Here's how the part is built. I have some questions about the finished solid (model axes, mm). Round coordinates to 2 decimals unless told otherwise and drop trailing zeros. Order: outer loops, then holes, each group sorted by start corner. A loop starts at its lowest first (then second) coordinate and runs counter-clockwise, first axis right, second up.
```python
from build123d import *

# Parameters (mm, degrees)
F0_W         = 73.972383514
F0_H         = 1.5005278401
F1_DEPTH     = 3.25
F2_R         = 1.375
F3_R         = 1.375
F4_T1_DEPTH  = 42.9737045288
F4_T3_DEPTH  = 0.5
F4_T5_DEPTH  = 97.1535263256
F4_T10_DEPTH = 1.375
F4_T16_DEPTH = 1.375
F4_T20_ANGLE = 62.6710528925
F4_T22_ANGLE = 62.6710528925


# Not quite as in the source:
# - a fillet or chamfer that OpenCascade refuses, or shapes differently, is made with other operations: its cross-section is extruded or revolved along the edge and cut away or added


with BuildPart() as f1:
    # F0 (on Top) → F1 (new body)
    with BuildSketch(Plane.XY):
        with BuildLine():
            Line((62.3850544982, 0), (62.3850544982, 8.25))
            Line((62.3850544982, 8.25), (-31.3309718274, 8.25))
            ThreePointArc((-31.3309718274, 8.25), (-35.6733794922, 7.0320400779), (-38.7489899112, 3.7334720175))
            Line((-38.7489899112, 3.7334720175), (-59.5149430004, -36.45))
            Line((-59.5149430004, -36.45), (-57.0939640871, -36.45))
            ThreePointArc((-57.0939640871, -36.45), (-52.4551081593, -35.0428751739), (-49.3797131513, -31.2957522588))
            Line((-49.3797131513, -31.2957522588), (-38.5501753509, -5.1542477412))
            ThreePointArc((-38.5501753509, -5.1542477412), (-35.474780343, -1.4071248261), (-30.8359244151, 0))
            Line((-30.8359244151, 0), (62.3850544982, 0))
        make_face()
        with Locations((14.1874579713, 4.9997360799)):
            Rectangle(F0_W, F0_H, mode=Mode.SUBTRACT)
    extrude(amount=F1_DEPTH)

    # F2
    f2_edges = [f1.edges().sort_by_distance(p)[0] for p in [
        (15.774565, 0, 3.25),
    ]]
    fillet(f2_edges, radius=F2_R)

    # F3
    f3_edges = [f1.edges().sort_by_distance(p)[0] for p in [
        (15.774565, 0, 0),
    ]]
    fillet(f3_edges, radius=F3_R)

    # F4: fillet of radius 1.375 on 2 edges, made by hand

    # F4_s2 → F4_t1 (cut)
    with BuildSketch(Plane(origin=(-6.6444578792, -12.8574588468, 0), x_dir=(0, 0, 1), z_dir=(-0.4590984452, -0.8883853993, 0))):
        with BuildLine():
            ThreePointArc((1.375, 36.1380680715), (0.4027281759, 35.7353398956), (0, 34.7630680715))
            Line((0, 34.7630680715), (0, 36.1380680715))
            Line((0, 36.1380680715), (1.375, 36.1380680715))
        make_face()
        with BuildLine():
            ThreePointArc((1.875, 36.1380680715), (2.8472718241, 35.7353398956), (3.25, 34.7630680715))
            Line((3.25, 34.7630680715), (3.25, 36.1380680715))
            Line((3.25, 36.1380680715), (1.875, 36.1380680715))
        make_face()
    extrude(amount=F4_T1_DEPTH, mode=Mode.SUBTRACT)

    # F4_s4 → F4_t3 (cut)
    with BuildSketch(Plane.XY.offset(1.375)):
        with BuildLine():
            ThreePointArc((-58.478150845, -34.4437396378), (-58.4310586584, -35.7900671304), (-57.256620921, -36.45))
            Line((-57.256620921, -36.45), (-59.5149430004, -36.45))
            Line((-59.5149430004, -36.45), (-58.478150845, -34.4437396378))
        make_face()
    extrude(amount=F4_T3_DEPTH, mode=Mode.SUBTRACT)

    # F4_s6 → F4_t5 (cut)
    with BuildSketch(Plane.YZ.offset(-31.3309718274)):
        with BuildLine():
            ThreePointArc((6.875, 3.25), (7.8472718241, 2.8472718241), (8.25, 1.875))
            Line((8.25, 1.875), (8.25, 3.25))
            Line((8.25, 3.25), (6.875, 3.25))
        make_face()
        with BuildLine():
            ThreePointArc((6.875, 0), (7.8472718241, 0.4027281759), (8.25, 1.375))
            Line((8.25, 1.375), (8.25, 0))
            Line((8.25, 0), (6.875, 0))
        make_face()
    extrude(amount=F4_T5_DEPTH, mode=Mode.SUBTRACT)


with BuildPart() as f4_tool8:
    # F4_s9 → F4_t10 (new body)
    with BuildSketch(Plane.XY.offset(1.875)):
        Polygon((-57.256620921, -35.075), (-58.478150845, -34.4437396378), (-59.5149430004, -36.45), (-57.256620921, -36.45), align=None)
    extrude(amount=F4_T10_DEPTH)

    # F4_s11 → F4_t12 (revolve, cut)
    with BuildSketch(Plane(origin=(-57.256620921, -35.075, 1.875), x_dir=(0.8541365363, 0.5200488221, 0), z_dir=(0.5200488221, -0.8541365363, 0))):
        with BuildLine():
            ThreePointArc((0, -1.375), (1.375, 0), (0, 1.375))
            Line((0, 1.375), (0, -1.375))
        make_face()
    revolve(axis=Axis((-57.256620921, -35.075, 1.875), (0, 0, 1)), mode=Mode.SUBTRACT)


with BuildPart() as f1_1:
    add(f1.part)

    # F4_t7: cut F4_tool8
    add(f4_tool8.part, mode=Mode.SUBTRACT)


with BuildPart() as f4_tool14:
    # F4_s15 → F4_t16 (new body)
    with BuildSketch(Plane.XY.offset(1.375)):
        Polygon((-57.256620921, -35.075), (-58.478150845, -34.4437396378), (-59.5149430004, -36.45), (-57.256620921, -36.45), align=None)
    extrude(amount=-F4_T16_DEPTH)

    # F4_s17 → F4_t18 (revolve, cut)
    with BuildSketch(Plane(origin=(-57.256620921, -35.075, 1.375), x_dir=(0.8541365363, 0.5200488221, 0), z_dir=(-0.5200488221, 0.8541365363, 0))):
        with BuildLine():
            ThreePointArc((0, -1.375), (1.375, 0), (0, 1.375))
            Line((0, 1.375), (0, -1.375))
        make_face()
    revolve(axis=Axis((-57.256620921, -35.075, 1.375), (0, 0, -1)), mode=Mode.SUBTRACT)


with BuildPart() as f1_2:
    add(f1_1.part)

    # F4_t13: cut F4_tool14
    add(f4_tool14.part, mode=Mode.SUBTRACT)

    # F4_s19 → F4_t20 (revolve, cut)
    with BuildSketch(Plane.YZ.offset(-31.3309718274)):
        with BuildLine():
            ThreePointArc((6.875, 3.25), (7.8472718241, 2.8472718241), (8.25, 1.875))
            Line((8.25, 1.875), (8.25, 3.25))
            Line((8.25, 3.25), (6.875, 3.25))
        make_face()
    revolve(axis=Axis((-31.3309718274, -0.1, 3.25), (0, 0, 1)), revolution_arc=F4_T20_ANGLE, mode=Mode.SUBTRACT)

    # F4_s21 → F4_t22 (revolve, cut)
    with BuildSketch(Plane.YZ.offset(-31.3309718274)):
        with BuildLine():
            ThreePointArc((6.875, 0), (7.8472718241, 0.4027281759), (8.25, 1.375))
            Line((8.25, 1.375), (8.25, 0))
            Line((8.25, 0), (6.875, 0))
        make_face()
    revolve(axis=Axis((-31.3309718274, -0.1, 0), (0, 0, 1)), revolution_arc=F4_T22_ANGLE, mode=Mode.SUBTRACT)


solid = f1_2.part
```
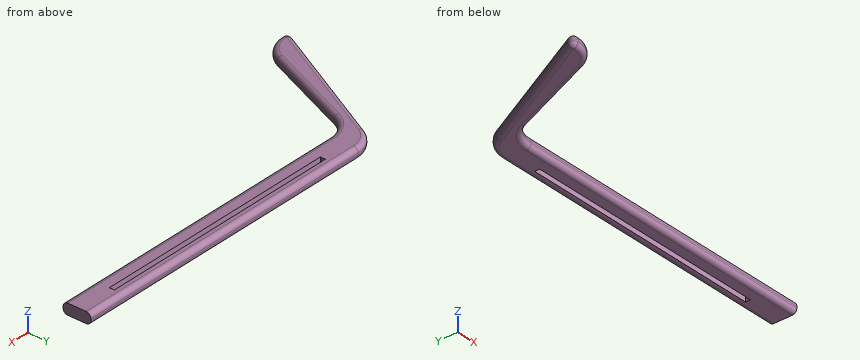
1. If we section it at B-B, the plane z = 2.55: Write out the boundary of the cut face in (x, y) (3 decimals), and give its area (3 significant figures).
Evaluation:
outline: (-58.321, -34.525) arc R1.198 ccw to (-57.257, -36.273) - (-57.094, -36.273) arc R8.173 ccw to (-49.543, -31.228) - (-38.714, -5.086) arc R8.527 cw to (-30.836, 0.177) - (62.385, 0.177) - (62.385, 8.073) - (-31.331, 8.073) arc R8.173 ccw to (-38.592, 3.652) - close; hole (-22.799, 4.249) - (51.174, 4.249) - (51.174, 5.75) - (-22.799, 5.75) - close
area: 888 mm2
2. I need wall thicknesses on probe 1 along Y at (x, z) = (17.5, 1.7); probe 2 along Y at (x, z) = (21.5, 0.3); probe 3 along Y at (x, z) = (56.5, 0.3). Which ranges of each line are inside material? Lowest first, please.
Evaluation:
probe 1: y = 0 to 4.25, 5.75 to 8.25
probe 2: y = 0.52 to 4.25, 5.75 to 7.73
probe 3: y = 0.52 to 7.73
3. If we section it at A-A, the plane x = 21.5: Write out the boundary of the cut face in (y, z) (3 decimals).
Evaluation:
outline: (0, 1.375) arc R1.375 ccw to (1.375, 0) - (4.249, 0) - (4.249, 3.25) - (1.375, 3.25) arc R1.375 ccw to (0, 1.875) - close; (5.75, 0) - (6.875, 0) arc R1.375 ccw to (8.25, 1.375) - (8.25, 1.875) arc R1.375 ccw to (6.875, 3.25) - (5.75, 3.25) - close
4. I'm going to push flat-ended pins straight in: P1, Ø1, axis at y = -20.5, z = 1.5, coming from the +X side; P2, Ø1, axis at x = 10.5, z = 0.5, coming from the -Y side; P3, Ø0.5, axis at y = 5, z = 2, coming from the -X side. Where does each tip first touch, or does it pass through?
Evaluation:
P1: stops at x = -44.7
P2: stops at y = 0.05
P3: stops at x = -38.12
